```python
from build123d import *

# Parameters (mm, degrees)
BOSS_EXTRUDE1_DEPTH     = 13.75
CUT_EXTRUDE1_DEPTH      = 52.529724432
CUT_EXTRUDE1_DEPTH_BACK = 52.529724432
SKETCH2_W               = 21
SKETCH2_H               = 5
BOSS_EXTRUDE2_START     = -1.5
BOSS_EXTRUDE2_DEPTH     = 1.5
SKETCH4_W               = 21
SKETCH4_H               = 5
CUT_EXTRUDE2_DEPTH      = 2
SKETCH5_W               = 22
SKETCH5_H               = 7
CUT_EXTRUDE3_DEPTH      = 2


with BuildPart() as part:
    # Sketch1 → Boss-Extrude1 (new, symmetric)
    with BuildSketch(Plane(origin=(0, 0, 0), x_dir=(1, 0, 0), z_dir=(0, 1, 0))):
        with BuildLine():
            Line((-26.5, 8), (-26.5, -8))
            ThreePointArc((-26.5, -8), (-22.399494937, -17.899494937), (-12.5, -22))
            Line((-12.5, -22), (12.5, -22))
            ThreePointArc((12.5, -22), (22.399494937, -17.899494937), (26.5, -8))
            Line((26.5, -8), (26.5, 8))
            ThreePointArc((26.5, 8), (22.399494937, 17.899494937), (12.5, 22))
            Line((12.5, 22), (-12.5, 22))
            ThreePointArc((-12.5, 22), (-22.399494937, 17.899494937), (-26.5, 8))
        make_face()
        with BuildLine():
            Line((12.5, -20), (-12.5, -20))
            ThreePointArc((-12.5, -20), (-20.985281374, -16.485281374), (-24.5, -8))
            Line((-24.5, -8), (-24.5, 8))
            ThreePointArc((-24.5, 8), (-20.985281374, 16.485281374), (-12.5, 20))
            Line((-12.5, 20), (12.5, 20))
            ThreePointArc((12.5, 20), (20.985281374, 16.485281374), (24.5, 8))
            Line((24.5, 8), (24.5, -8))
            ThreePointArc((24.5, -8), (20.985281374, -16.485281374), (12.5, -20))
        make_face(mode=Mode.SUBTRACT)
    extrude(amount=BOSS_EXTRUDE1_DEPTH, both=True)

    # Sketch2 → Cut-Extrude1 (cut, two sides: drawn at the far end of the back side and taken through both)
    with BuildSketch(Plane.XY.offset(-20).offset(-CUT_EXTRUDE1_DEPTH_BACK)):
        with Locations((0, 9.5)):
            Rectangle(SKETCH2_W, SKETCH2_H)
    extrude(amount=CUT_EXTRUDE1_DEPTH + CUT_EXTRUDE1_DEPTH_BACK, mode=Mode.SUBTRACT)

    # Sketch3 → Boss-Extrude2 (add)
    with BuildSketch(Plane.XZ.offset(13.75).offset(BOSS_EXTRUDE2_START)):
        with BuildLine():
            Line((-12.5, -22), (12.5, -22))
            ThreePointArc((12.5, -22), (22.399494937, -17.899494937), (26.5, -8))
            Line((26.5, -8), (26.5, 8))
            ThreePointArc((26.5, 8), (22.399494937, 17.899494937), (12.5, 22))
            Line((12.5, 22), (-12.5, 22))
            ThreePointArc((-12.5, 22), (-22.399494937, 17.899494937), (-26.5, 8))
            Line((-26.5, 8), (-26.5, -8))
            ThreePointArc((-26.5, -8), (-22.399494937, -17.899494937), (-12.5, -22))
        make_face()
    extrude(amount=BOSS_EXTRUDE2_DEPTH)

    # Sketch4 → Cut-Extrude2 (cut)
    with BuildSketch(Plane(origin=(0, 0, -22), x_dir=(-1, 0, 0), z_dir=(0, 0, -1))):
        with Locations((0, -7.5)):
            Rectangle(SKETCH4_W, SKETCH4_H)
    extrude(amount=-CUT_EXTRUDE2_DEPTH, mode=Mode.SUBTRACT)

    # Sketch5 → Cut-Extrude3 (cut)
    with BuildSketch(Plane(origin=(0, -12.25, 0), x_dir=(-1, 0, 0), z_dir=(0, 1, 0))):
        with Locations((0, -15.5)):
            Rectangle(SKETCH5_W, SKETCH5_H)
    extrude(amount=-CUT_EXTRUDE3_DEPTH, mode=Mode.SUBTRACT)


solid = part.part
```
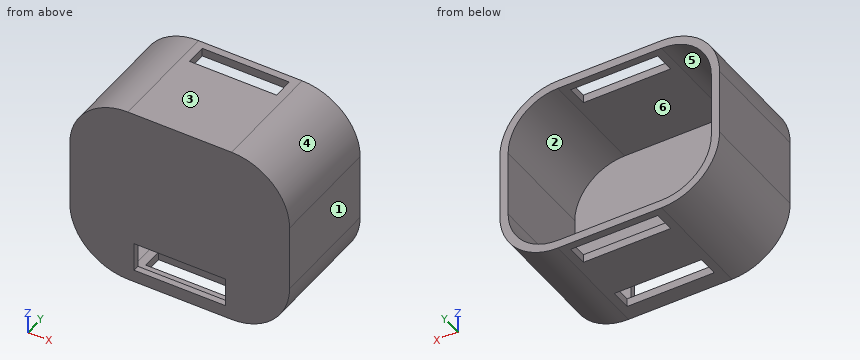
Design review of the part built by this model. Coordinates are the model's own, in mm. Face numbers are marked on the shaded views. A direction names the side the tool comes from. Round coordinates to 2 decimals unless told otherwise and drop trailing zeros. Write each loop counter-clockwise with the first axis right and the second up, starting at its lowest first coordinate (ties: lowest second). Pieces come first, ordered by that corner, then holes.
Item 1: For probe 1 along Z at (x, y) = (-3.5, 1.75); probe 2 along X at (y, z) = (-2.5, -2); probe 3 along Y at (x, z) = (-6, 10.5), list the stretches that pass through material, from the lowest coordinate up.
Item 2: We need section A-A on y = 9.75. Write out the cut boundary in (x, z).
Item 3: We need section B-B on x = -9. Write out the cut boundary in (y, z).
Item 4: The part is to be moulded in two halves that separate along X. For the marked faces 3, 4, 5 and 6, say which applies: +X half, -X half, draft (parallel to the pull), parting line (faces both ways), or undercut.
Item 5: We need section C-C on y = 5. Write out the cut boundary in (x, z), and give its area (3 significant figures).
Item 6: For the marked faces 1 and 2, list the 3-axis set-ups (+Z, -Z, +X, -X, +Y, -Y) from which the entire face can be reached by the end or side of a thin tool; tool diameter is ignored.
Item 7: We need section D-D on z = 0. Write out the cut boundary in (x, y).
Item 8: Clearance check with flat-ended pins moving along their axes: pin 1 Ø1.5 at (x, z) = (-14.5, -15.5) entering from +Y; pin 2 Ø1.6 at (y, z) = (9, -20.5) entering from -X; pin 3 Ø0.6 at (y, z) = (8.5, 21) entering from -X. State where each tip first meets the part, or that it passes through.
Returned:
1. probe 1: z = -22 to -20, 20 to 22
1. probe 2: x = -26.5 to -24.5, 24.5 to 26.5
1. probe 3: y = -13.75 to -12.25
2. outline: (-26.5, -8) arc R14 ccw to (-12.5, -22) - (-10.5, -22) - (-10.5, -20) - (-12.5, -20) arc R12 cw to (-24.5, -8) - (-24.5, 8) arc R12 cw to (-12.5, 20) - (-10.5, 20) - (-10.5, 22) - (-12.5, 22) arc R14 ccw to (-26.5, 8) - close; (10.5, -22) - (12.5, -22) arc R14 ccw to (26.5, -8) - (26.5, 8) arc R14 ccw to (12.5, 22) - (10.5, 22) - (10.5, 20) - (12.5, 20) arc R12 cw to (24.5, 8) - (24.5, -8) arc R12 cw to (12.5, -20) - (10.5, -20) - close
3. outline: (-13.75, -22) - (-10, -22) - (-10, -20) - (-12.25, -20) - (-12.25, -19) - (-13.75, -19) - close; (-13.75, -12) - (-12.25, -12) - (-12.25, 20) - (7, 20) - (7, 22) - (-13.75, 22) - close; (-5, -22) - (7, -22) - (7, -20) - (-5, -20) - close; (12, -22) - (13.75, -22) - (13.75, -20) - (12, -20) - close; (12, 20) - (13.75, 20) - (13.75, 22) - (12, 22) - close
4. face 3: draft
4. face 4: +X half
4. face 5: undercut
4. face 6: undercut
5. outline: (-26.5, -8) arc R14 ccw to (-12.5, -22) - (12.5, -22) arc R14 ccw to (26.5, -8) - (26.5, 8) arc R14 ccw to (12.5, 22) - (-12.5, 22) arc R14 ccw to (-26.5, 8) - close; hole (-24.5, -8) arc R12 ccw to (-12.5, -20) - (12.5, -20) arc R12 ccw to (24.5, -8) - (24.5, 8) arc R12 ccw to (12.5, 20) - (-12.5, 20) arc R12 ccw to (-24.5, 8) - close
5. area: 327 mm2
6. face 1: +Z, -Z, +X, +Y, -Y
6. face 2: +Y
7. outline: (-26.5, -13.75) - (26.5, -13.75) - (26.5, 13.75) - (24.5, 13.75) - (24.5, -12.25) - (-24.5, -12.25) - (-24.5, 13.75) - (-26.5, 13.75) - close
8. pin 1: stops at y = -12.25
8. pin 2: stops at x = -20.19
8. pin 3: stops at x = -18.39
